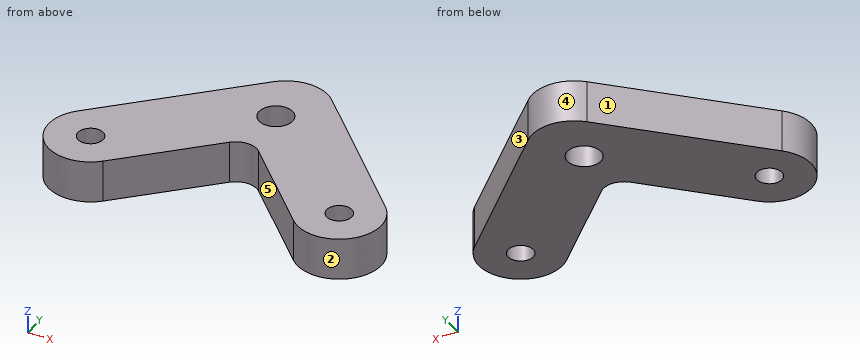
from build123d import *

# Parameters (mm, degrees)
EXTRUDE_1_DEPTH     = 10
SKETCH_2_R          = 4
SKETCH_2_R_2        = 3
CUT_EXTRUDE_1_DEPTH = 10
FILLET_1_R          = 5


with BuildPart() as part:
    # 草图1 → 凸台-拉伸1 (new body)
    with BuildSketch(Plane.XY):
        with BuildLine():
            Line((-7.071067812, 11.264774836), (-37.071067812, -18.735225164))
            ThreePointArc((-37.071067812, -18.735225164), (-37.071067812, -32.877360787), (-22.928932188, -32.877360787))
            Line((-22.928932188, -32.877360787), (0, -9.948428599))
            Line((0, -9.948428599), (22.928932188, -32.877360787))
            ThreePointArc((22.928932188, -32.877360787), (37.071067812, -32.877360787), (37.071067812, -18.735225164))
            Line((37.071067812, -18.735225164), (7.071067812, 11.264774836))
            ThreePointArc((7.071067812, 11.264774836), (0, 14.193707024), (-7.071067812, 11.264774836))
        make_face()
    extrude(amount=EXTRUDE_1_DEPTH)

    # 草图2 → 切除-拉伸1 (cut)
    with BuildSketch(Plane.XY.offset(10)):
        Circle(SKETCH_2_R)
        with Locations((-30, -25.806292976)):
            Circle(SKETCH_2_R_2)
        with Locations((30, -25.806292976)):
            Circle(SKETCH_2_R_2)
    extrude(amount=-CUT_EXTRUDE_1_DEPTH, mode=Mode.SUBTRACT)

    # 圆角1
    fillet_1_edges = [part.edges().sort_by_distance(p)[0] for p in [
        (0, -9.948428599, 5),
    ]]
    fillet(fillet_1_edges, radius=FILLET_1_R)


solid = part.part
The model under review builds one solid part; all positions refer to its coordinate system, in mm. Face numbers are marked on the shaded views. A direction names the side the tool comes from. Round coordinates to 2 decimals unless told otherwise and drop trailing zeros. Loops run counter-clockwise (first coordinate to the right, second up) from the corner with the lowest first, then second, coordinate; pieces in that order, holes last. Notation, with made-up numbers: (12.25, 25) -> (41.25, 25) arc R7 ccw to (41.25, 37) -> close; hole circle Ø7 at (44.5, 1). An arc over 180 degrees is marked (long way). Return JSON: item names as keys, results as strings.
(1) Add section A-A on x = 0. Write out the cut boundary in (y, z), plus the area to 3 significant figures.
Solved:
{"outline": "(-12.02, 0) -> (-4, 0) -> (-4, 10) -> (-12.02, 10) -> close; (4, 0) -> (14.19, 0) -> (14.19, 10) -> (4, 10) -> close", "area": "182 mm2"}
(2) For the marked faces 4 and 5, list the 3-axis set-ups (+Z, -Z, +X, -X, +Y, -Y) from which the entire face can be reached by the end or side of a thin tool; tool diameter is ignored.
Solved:
{"face 4": "+Z, -Z, +Y", "face 5": "+Z, -Z, -Y"}
(3) For pin 1 (6 mm diameter, centred on x = 15.5, z = 1, fed in from -Y); pin 2 (5 mm diameter, centred on y = -27, z = 2, fed in from -X); pin 3 (6 mm diameter, centred on x = 8.5, z = 2, fed in from +Y); pin 4 (5 mm diameter, centred on x = 30, y = -25.81, fed in from -Z), all flat-tipped, find the tip position at first contact; note any pin that passes through.
Solved:
{"pin 1": "y = -28.45", "pin 2": "x = -40", "pin 3": "y = 12.55", "pin 4": "through"}
(4) The part is to be moulded in two halves that separate along X. For the marked faces 1, 2 and 3, say which applies: released by +X, released by -X, zero draft, split by the parting line, or undercut.
Solved:
{"face 1": "released by -X", "face 2": "undercut", "face 3": "released by +X"}
(5) Add section B-B on y = -30. Write out the cut boundary in (x, z).
Solved:
{"outline": "(-39.08, 0) -> (-20.05, 0) -> (-20.05, 10) -> (-39.08, 10) -> close; (20.05, 0) -> (39.08, 0) -> (39.08, 10) -> (20.05, 10) -> close"}
(6) For line 1 (X direction, y = -26, z = 3.75); line 2 (Y direction, x = 0, z = 4); line 3 (X direction, y = -26.5, z = 3.25), list the stretches that pass through material, from the lowest coordinate up.
Solved:
{"line 1": "-40 to -32.99, -27.01 to -16.05, 16.05 to 27.01, 32.99 to 40", "line 2": "-12.02 to -4, 4 to 14.19", "line 3": "-39.98 to -32.92, -27.08 to -16.55, 16.55 to 27.08, 32.92 to 39.98"}
(7) Add section C-C on z = 6. Write out the cut boundary in (x, y), plus the area to 3 significant figures.
Solved:
{"outline": "(-37.07, -18.74) arc R10 ccw to (-22.93, -32.88) -> (-3.54, -13.48) arc R5 cw to (3.54, -13.48) -> (22.93, -32.88) arc R10 ccw to (37.07, -18.74) -> (7.07, 11.26) arc R10 ccw to (-7.07, 11.26) -> close; hole circle Ø6 at (-30, -25.81); hole circle Ø8 at (0, 0); hole circle Ø6 at (30, -25.81)", "area": "1,890 mm2"}
(8) Add section D-D on y = 8.5. Write out the cut boundary in (x, z).
Solved:
{"outline": "(-9.84, 0) -> (9.84, 0) -> (9.84, 10) -> (-9.84, 10) -> close"}
